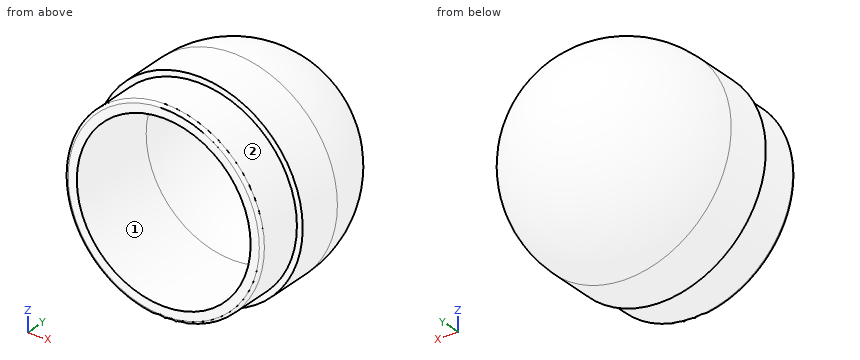
from build123d import *


with BuildPart() as part:
    # Sketch2 → Revolve1 (revolve)
    with BuildSketch(Plane.XY):
        with BuildLine():
            Line((47.625, 0), (52.3875, 0))
            ThreePointArc((52.3875, 0), (53.510032015, 0.464967985), (53.975, 1.5875))
            Line((53.975, 1.5875), (53.975, 25.4))
            Line((53.975, 25.4), (57.15, 25.4))
            Line((57.15, 25.4), (57.15, 50.8))
            ThreePointArc((57.15, 50.8), (40.411152545, 91.211152545), (0, 107.95))
            Line((0, 107.95), (0, 98.425))
            ThreePointArc((0, 98.425), (33.675960454, 84.475960454), (47.625, 50.8))
            Line((47.625, 50.8), (47.625, 0))
        make_face()
    revolve(axis=Axis((0, 98.425, 0), (0, 1, 0)))


solid = part.part
Could you check a few things on this model? Use its own coordinates, in mm. Face numbers are marked on the shaded views. Give positions to 0.01 mm unless a question says otherwise; leave off trailing zeros. Order: outer loops, then holes, each group sorted by start corner. A loop starts at its lowest first (then second) coordinate and runs counter-clockwise, first axis right, second up. Notation, with made-up numbers: (84, 39.5) -> (141, 39.5) arc R25 ccw to (141, 63.5) -> close; hole circle Ø5 at (63.5, -29.5). An arc over 180 degrees is marked (long way). Answer in a Markdown table with one row per item. Add a question column.
Item 1: I'm going to push flat-ended pins straight in: P1, Ø12, axis at x = -39, z = 35.5, coming from the +Y side; P2, Ø12, axis at x = 17.5, z = 14.5, coming from the +Y side; P3, Ø6, axis at x = 32.5, y = 17.5, coming from the -Z side. Where does each tip first touch, or does it pass through?
Item 2: We'd pull the mould along X, two halves only. Please class the marked faces 1 and 2: pulls with the +X half, pulls with the -X half, needs draft (parallel to the pull), parting line crosses it, or undercut.
Item 3: Please list where these lines run through material, in increasing order: probe 1 along X at (y, z) = (25.5, 0) (3 decimals); probe 2 along Z at (x, y) = (0, 20) (3 decimals).
Item 4: Imagine slicing it at C-C (y = 43). List the corners of the cut face in (x, z) for me (3 decimals).
Item 5: Imagine slicing it at D-D (y = 21). List the corners of the cut face in (x, z) for me (3 decimals).
Result:
| question | item | result |
|---|---|---|
| 1 | P1 | y = 83.69 |
| 1 | P2 | y = 105.45 |
| 1 | P3 | z = -45.2 |
| 2 | face 1 | undercut |
| 2 | face 2 | parting line crosses it |
| 3 | probe 1 | -57.15 to -47.625, 47.625 to 57.15 |
| 3 | probe 2 | -53.975 to -47.625, 47.625 to 53.975 |
| 4 | outline | circle Ø114.3 at (0, 0); hole circle Ø95.25 at (0, 0) |
| 5 | outline | circle Ø107.95 at (0, 0); hole circle Ø95.25 at (0, 0) |
